Geometry: final body of the model. Coordinates: model frame, mm. Give positions to 0.01 mm unless a question says otherwise; leave off trailing zeros. Loops run counter-clockwise (first coordinate to the right, second up) from the corner with the lowest first, then second, coordinate; pieces in that order, holes last. Notation, with made-up numbers: (25, 78.25) - (68, 78.25) arc R15 cw to (68, 89.25) - close; hole circle Ø8 at (14.5, 78). An arc over 180 degrees is marked (long way). Answer in a Markdown table with one row per item.
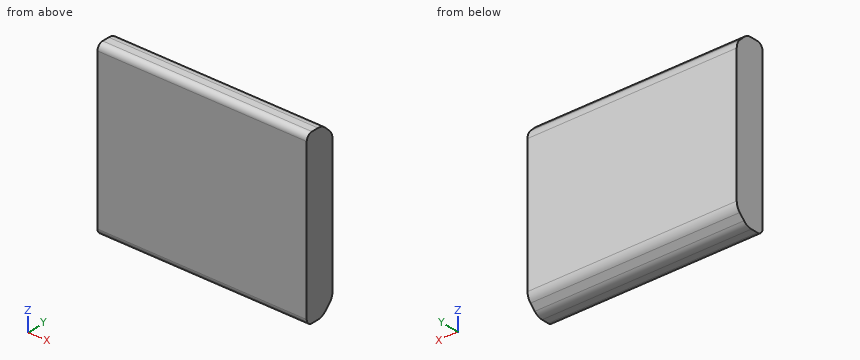
from build123d import *

# Parameters (mm, degrees)
BOSS_EXTRUDE1_START = -35
BOSS_EXTRUDE1_DEPTH = 69


with BuildPart() as part:
    # Sketch2 → Boss-Extrude1 (new body)
    with BuildSketch(Plane(origin=(0, 0, 0), x_dir=(0, 0, -1), z_dir=(1, 0, 0)).offset(BOSS_EXTRUDE1_START)):
        with BuildLine():
            Line((28, -13.656854249), (28, -16))
            ThreePointArc((28, -16), (27.414213562, -17.414213562), (26, -18))
            Line((26, -18), (-26, -18))
            ThreePointArc((-26, -18), (-27.414213562, -17.414213562), (-28, -16))
            Line((-28, -16), (-28, -13.656854249))
            ThreePointArc((-28, -13.656854249), (-27.69551813, -12.12612052), (-26.828427125, -10.828427125))
            Line((-26.828427125, -10.828427125), (-25.171572875, -9.171572875))
            ThreePointArc((-25.171572875, -9.171572875), (-23.87387948, -8.30448187), (-22.343145751, -8))
            Line((-22.343145751, -8), (22.343145751, -8))
            ThreePointArc((22.343145751, -8), (23.87387948, -8.30448187), (25.171572875, -9.171572875))
            Line((25.171572875, -9.171572875), (26.828427125, -10.828427125))
            ThreePointArc((26.828427125, -10.828427125), (27.69551813, -12.12612052), (28, -13.656854249))
        make_face()
    extrude(amount=BOSS_EXTRUDE1_DEPTH)


solid = part.part
Q1. Material intervals for line 1 along Z through (x, y) = (25, -16.25); line 2 along Z through (x, y) = (28.5, -10.75); line 3 along Y through (x, z) = (-20.5, 23), sorted ascending.
Check values:
| item | result |
|---|---|
| line 1 | -27.98 to 27.98 |
| line 2 | -26.75 to 26.75 |
| line 3 | -18 to -8.05 |
Q2. First-contact query: pin 1 (3 mm diameter, centred on x = -17.5, y = -9.5, fed in from +Z); pin 2 (3 mm diameter, centred on x = -3.5, y = -10.5, fed in from +Z). Flat tips, straight axial feed; report the tip coordinate or a pass-through.
Check values:
| item | result |
|---|---|
| pin 1 | z = 26.99 |
| pin 2 | z = 27.64 |
Q3. Cut plane A-A (x = 19). Output: boundary loops of the cut face in (y, z).
Check values:
| item | result |
|---|---|
| outline | (-18, -26) arc R2 ccw to (-16, -28) - (-13.66, -28) arc R4 ccw to (-10.83, -26.83) - (-9.17, -25.17) arc R4 ccw to (-8, -22.34) - (-8, 22.34) arc R4 ccw to (-9.17, 25.17) - (-10.83, 26.83) arc R4 ccw to (-13.66, 28) - (-16, 28) arc R2 ccw to (-18, 26) - close |
